Answer from the drawing. Dimensions are ordinates in mm from the lowest x, y and z of the part. Round coordinates to 2 decimals unless told otherwise and drop trailing zeros. Write each loop counter-clockwise with the first axis right and the second up, starting at its lowest first coordinate (ties: lowest second). Pieces come first, ordered by that corner, then holes. Notation, with made-up numbers: (-40, 29.5) - (-27, 29.5) arc R19 ccw to (-27, 63.5) - close; hole circle Ø11 at (35, 53). An arc over 180 degrees is marked (long way). Answer in a Markdown table with one row per item.
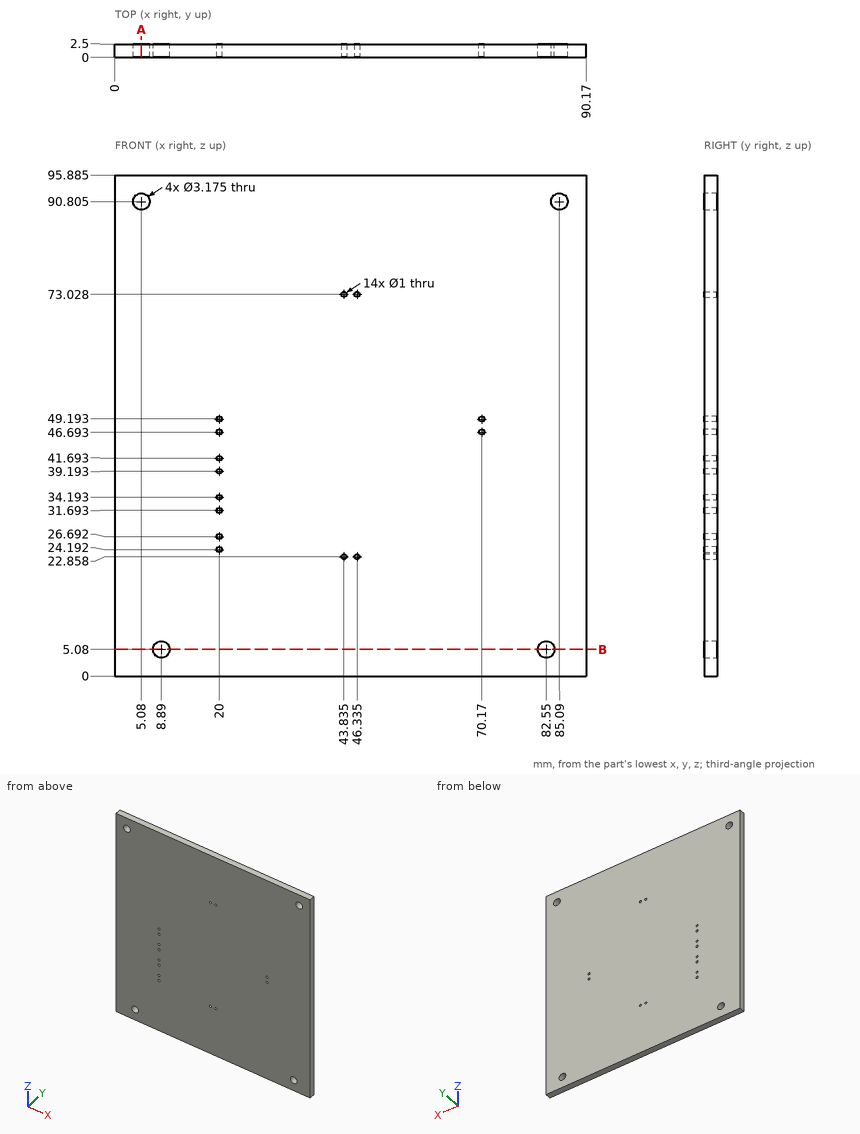
(1) A flat-ended cylindrical pin translates along its axis: pin 1 (1 mm diameter, centred on x = 56, y = 0.5, fed in from -Z). Find the tip coordinate at first contact, or state that the pin passes through.
Checked values:
| item | result |
|---|---|
| pin 1 | stops at z = 0 |
(2) Section B-B (z = 5.08) is taken. Give the vertices of the cut face in (x, y).
Checked values:
| item | result |
|---|---|
| outline | (0, 0) - (7.3, 0) - (7.3, 2.5) - (0, 2.5) - close; (10.48, 0) - (80.96, 0) - (80.96, 2.5) - (10.48, 2.5) - close; (84.14, 0) - (90.17, 0) - (90.17, 2.5) - (84.14, 2.5) - close |
(3) Section A-A (x = 5.08) is taken. Give the vertices of the cut face in (y, z) (1 decimal).
Checked values:
| item | result |
|---|---|
| outline | (0, 0) - (2.5, 0) - (2.5, 89.2) - (0, 89.2) - close; (0, 92.4) - (2.5, 92.4) - (2.5, 95.9) - (0, 95.9) - close |
(4) Find the intervals of material crossed by line 1 (X direction, y = 1.8, z = 5.08); line 2 (X direction, y = 0.5, z = 89.5) (1 decimal); line 3 (Z direction, x = 9, y = 1.9) (1 decimal), in increasing order.
Checked values:
| item | result |
|---|---|
| line 1 | x = 0 to 7.3, 10.48 to 80.96, 84.14 to 90.17 |
| line 2 | x = 0 to 4.2, 6 to 84.2, 86 to 90.2 |
| line 3 | z = 0 to 3.5, 6.7 to 95.9 |
